The listing builds one solid part. Answer for the finished solid, in the listing's coordinates (mm). A direction names the side the tool comes from. Give positions to 0.01 mm unless a question says otherwise; leave off trailing zeros. Return JSON: item names as keys, results as strings.
from build123d import *

# Parameters (mm, degrees)
SKETCH1_W           = 203.2
SKETCH1_H           = 254
BOSS_EXTRUDE1_DEPTH = 5.08
FILLET1_SIZE        = 64.219666667
FILLET1_SIZE_2      = 101.6
SKETCH14_W          = 5.08
SKETCH14_H          = 12.7
CUT_EXTRUDE2_DEPTH  = 326.318377121
CUT_EXTRUDE3_DEPTH  = 326.318377121


with BuildPart() as part:
    # Sketch1 → Boss-Extrude1 (new body)
    with BuildSketch(Plane.XY):
        with Locations((101.6, 127)):
            Rectangle(SKETCH1_W, SKETCH1_H)
    extrude(amount=BOSS_EXTRUDE1_DEPTH)

    # Fillet1
    # a fillet whose section is not a circle: 101.6, 64.219666667 mm, written as the material it takes off along each edge
    with BuildSketch(Plane(origin=(203.2, 254, -254), x_dir=(0, -1, 0), z_dir=(0, 0, 1))) as fillet1_piece_1:
        with BuildLine():
            Bezier((FILLET1_SIZE, 0), (0, 0), (0, -FILLET1_SIZE_2), weights=[1, 1, 1])
            Line((0, -FILLET1_SIZE_2), (0, 0))
            Line((0, 0), (FILLET1_SIZE, 0))
        make_face()
    extrude(amount=513.08, mode=Mode.SUBTRACT)
    with BuildSketch(Plane(origin=(0, 254, -254), x_dir=(1, 0, 0), z_dir=(0, 0, 1)), Plane(origin=(203.2, 0, -254), x_dir=(-1, 0, 0), z_dir=(0, 0, 1))) as fillet1_piece_2:
        with BuildLine():
            Bezier((FILLET1_SIZE_2, 0), (0, 0), (0, -FILLET1_SIZE), weights=[1, 1, 1])
            Line((0, -FILLET1_SIZE), (0, 0))
            Line((0, 0), (FILLET1_SIZE_2, 0))
        make_face()
    extrude(amount=513.08, mode=Mode.SUBTRACT)
    with BuildSketch(Plane(origin=(0, 0, -254), x_dir=(1, 0, 0), z_dir=(0, 0, 1))) as fillet1_piece_3:
        with BuildLine():
            Bezier((FILLET1_SIZE_2, 0), (0, 0), (0, FILLET1_SIZE), weights=[1, 1, 1])
            Line((0, FILLET1_SIZE), (0, 0))
            Line((0, 0), (FILLET1_SIZE_2, 0))
        make_face()
    extrude(amount=513.08, mode=Mode.SUBTRACT)

    # Sketch14 → Cut-Extrude2 (cut, through all)
    with BuildSketch(Plane.XY.offset(5.08)):
        with Locations((101.6, 234.95)):
            Rectangle(SKETCH14_W, SKETCH14_H)
        with Locations((101.6, 19.05)):
            Rectangle(SKETCH14_W, SKETCH14_H)
    extrude(amount=-CUT_EXTRUDE2_DEPTH, mode=Mode.SUBTRACT)

    # Sketch13 → Cut-Extrude3 (cut, through all)
    with BuildSketch(Plane.XY.offset(5.08)):
        Polygon((25.4, 222.25), (20.32, 222.25), (20.32, 209.55), (25.4, 209.55), (25.4, 215.9), align=None)
        Polygon((177.8, 215.9), (177.8, 222.25), (182.88, 222.25), (182.88, 209.55), (177.8, 209.55), align=None)
        Polygon((177.8, 38.1), (177.8, 44.45), (182.88, 44.45), (182.88, 31.75), (177.8, 31.75), align=None)
        Polygon((25.4, 38.1), (25.4, 44.45), (20.32, 44.45), (20.32, 31.75), (25.4, 31.75), align=None)
        Polygon((187.96, 168.275), (187.96, 165.735), (195.58, 165.735), (195.58, 170.815), (187.96, 170.815), align=None)
        Polygon((187.96, 85.725), (187.96, 88.265), (195.58, 88.265), (195.58, 83.185), (187.96, 83.185), align=None)
        Polygon((15.24, 168.275), (15.24, 170.815), (7.62, 170.815), (7.62, 165.735), (15.24, 165.735), align=None)
        Polygon((15.24, 85.725), (15.24, 88.265), (7.62, 88.265), (7.62, 83.185), (15.24, 83.185), align=None)
    extrude(amount=-CUT_EXTRUDE3_DEPTH, mode=Mode.SUBTRACT)


solid = part.part
Item 1: Flat-ended cylindrical pins translate along their axes: P1, Ø1.5, axis at y = 20.5, z = 2.5, coming from the -X side; P2, Ø1.5, axis at x = 179.5, z = 2, coming from the +Y side; P3, Ø1.5, axis at y = 217.5, z = 3, coming from the -X side. Find the tip coordinate at first contact, or state that the pin passes through.
Answer below:
{"P1": "stops at x = 18.33", "P2": "stops at y = 237.33", "P3": "stops at x = 5.77"}
Item 2: A cutting plane is placed at A-A on z = 3.1. Give the number of separate pieces and of enclosed holes in the cut face, then the cut area to 3 significant figures.
Answer below:
{"separate pieces": "1", "enclosed holes": "10", "area": "46,700 mm²"}
Item 3: Consider L1, parallel to Y at x = 100, z = 4.4; L2, parallel to Y at x = 10, z = 4.2 (1 decimal); L3, parallel to X at y = 39, z = 4.45. Determine where each line is inside the solid, lowest interval first.
Answer below:
{"L1": "y = 0 to 12.7, 25.4 to 228.6, 241.3 to 254", "L2": "y = 30.2 to 83.2, 88.3 to 165.7, 170.8 to 223.8", "L3": "x = 4.95 to 20.32, 25.4 to 177.8, 182.88 to 198.25"}
Item 4: For faces 1 (the face through (7.62, 168, 3)), 2 (the face through (100, 129, 5.08)), determine the directions among +Z, -Z, +X, -X, +Y, -Y from which every point of the face is accessible in a straight line to the end or side of a thin tool.
Answer below:
{"face 1": "+Z, -Z", "face 2": "+Z, +X, -X, +Y, -Y"}
Item 5: The mould has two halves that part along X. Classify faces 3 (the face through (100, 129, 0)), 4 (the face through (20.32, 38, 3)): +X half, -X half, draft (parallel to the pull), parting line (faces both ways), or undercut.
Answer below:
{"face 3": "draft", "face 4": "undercut"}
